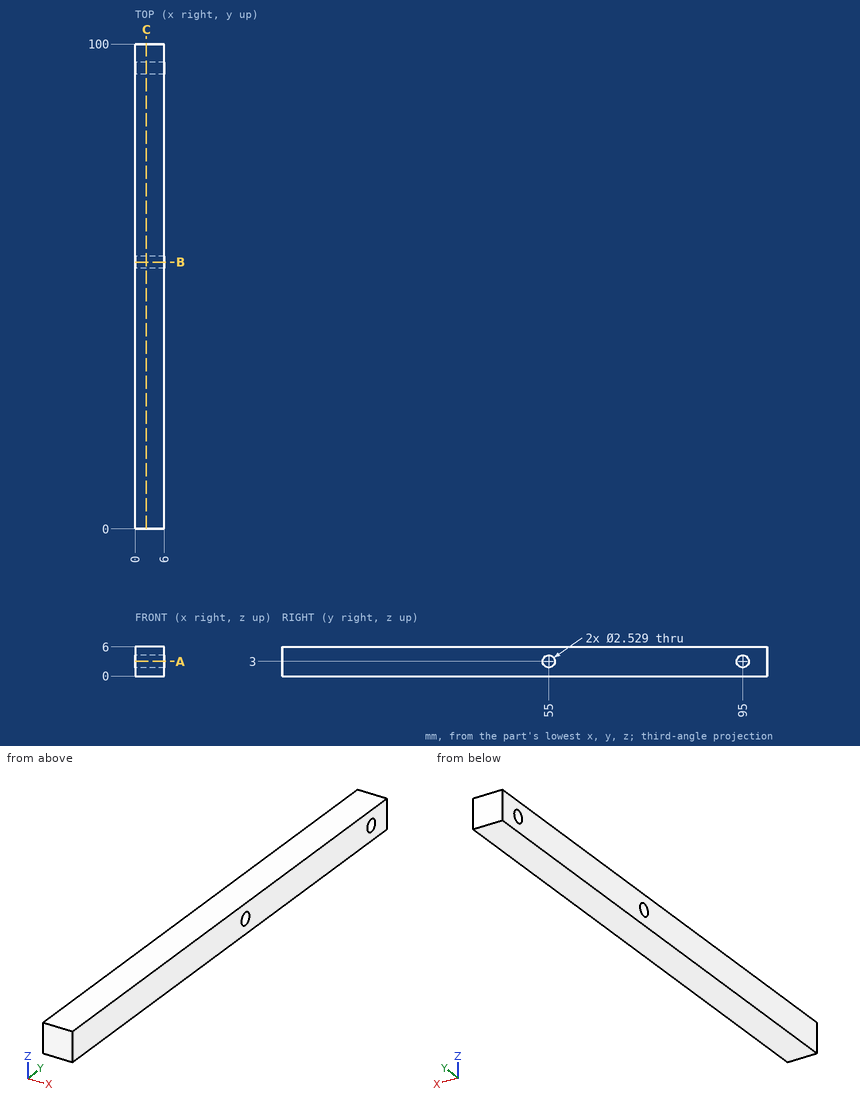
The drawing under review shows one solid part. Ordinate dimensions are in mm from its lowest x, y, z. Round coordinates to 2 decimals unless told otherwise and drop trailing zeros. Order: outer loops, then holes, each group sorted by start corner. A loop starts at its lowest first (then second) coordinate and runs counter-clockwise, first axis right, second up. Notation, with made-up numbers: (84, -10) -> (138, -10) arc R22 cw to (138, 18) -> close; hole circle Ø3 at (-11.75, 54.25). An arc over 180 degrees is marked (long way). Use a Markdown table: item, result.
Item 1: Take a section at C-C (x = 2.35). State the section outline as (y, z) points.
Resolved:
| item | result |
|---|---|
| outline | (0, 0) -> (100, 0) -> (100, 6) -> (0, 6) -> close; hole circle Ø2.53 at (55, 3); hole circle Ø2.53 at (95, 3) |
Item 2: Take a section at B-B (y = 55). State the section outline as (x, z) points, plus the area to 3 significant figures.
Resolved:
| item | result |
|---|---|
| outline | (0, 0) -> (6, 0) -> (6, 1.74) -> (0, 1.74) -> close; (0, 4.26) -> (6, 4.26) -> (6, 6) -> (0, 6) -> close |
| area | 20.8 mm² |
Item 3: For line 1 along Y through (x, z) = (1.5, 3); line 2 along Y through (x, z) = (0.85, 3.35); line 3 along Z through (x, y) = (2.3, 95), list the stretches that pass through material, from the lowest coordinate up. Write a range as [from, to].
Resolved:
| item | result |
|---|---|
| line 1 | y = [0, 53.74], [56.26, 93.74], [96.26, 100] |
| line 2 | y = [0, 53.78], [56.22, 93.78], [96.22, 100] |
| line 3 | z = [0, 1.74], [4.26, 6] |
Item 4: Take a section at A-A (z = 3). State the section outline as (x, y) points.
Resolved:
| item | result |
|---|---|
| outline | (0, 0) -> (6, 0) -> (6, 53.74) -> (0, 53.74) -> close; (0, 56.26) -> (6, 56.26) -> (6, 93.74) -> (0, 93.74) -> close; (0, 96.26) -> (6, 96.26) -> (6, 100) -> (0, 100) -> close |
